Source: CAD feature listing. Evaluate the final solid. Frame: model axes, mm. A direction names the side the tool comes from. Round coordinates to 2 decimals unless told otherwise and drop trailing zeros. Order: outer loops, then holes, each group sorted by start corner. A loop starts at its lowest first (then second) coordinate and runs counter-clockwise, first axis right, second up. Notation, with made-up numbers: M 13.25,55.25 L 22.25,55.25 A8 ccw 22.25,60.25 Z; hole C 47.25,41.5 d7. An arc over 180 degrees is marked long. Answer in a Markdown table with one row per item. Add a question column.
```python
from build123d import *

# Parameters (mm, degrees)
SKETCH1_W                   = 30
SKETCH1_H                   = 30
BOSS_EXTRUDE1_DEPTH         = 5
SKETCH2_W                   = 1
SKETCH2_H                   = 30
BOSS_EXTRUDE2_DEPTH         = 4
LPATTERN1_COUNT             = 2
LPATTERN1_PITCH             = 10
CIRPATTERN1_COUNT           = 2
CIRPATTERN1_ANGLE           = 90
CIRPATTERN1_COPY_1_SKETCH_W = 1
CIRPATTERN1_COPY_1_SKETCH_H = 30
CIRPATTERN1_COPY_1_DEPTH    = 4
CUT_EXTRUDE2_DEPTH          = 22.794494718
CUT_EXTRUDE2_DEPTH_BACK     = 22.794494718
SKETCH4_R                   = 5
SKETCH8_W                   = 30
SKETCH8_H                   = 30
BOSS_EXTRUDE3_DEPTH         = 5
CUT_EXTRUDE3_DEPTH          = 5


# Read off the part's stored shape, not the designer's step: Cut-Extrude3
with BuildPart() as part:
    # Sketch1 → Boss-Extrude1 (new body)
    with BuildSketch(Plane(origin=(0, 0, 0), x_dir=(1, 0, 0), z_dir=(0, 1, 0))):
        Rectangle(SKETCH1_W, SKETCH1_H)
    extrude(amount=BOSS_EXTRUDE1_DEPTH)

    # Sketch2 → Boss-Extrude2 (add)
    with BuildSketch(Plane(origin=(0, 5, 0), x_dir=(1, 0, 0), z_dir=(0, 1, 0))):
        with Locations((-5, 0)):
            Rectangle(SKETCH2_W, SKETCH2_H)
    boss_extrude2 = extrude(amount=BOSS_EXTRUDE2_DEPTH)

    # LPattern1: Boss-Extrude2 ×2
    with Locations(*[(i * LPATTERN1_PITCH, 0, 0) for i in range(1, LPATTERN1_COUNT)]):
        add(boss_extrude2)

    # CirPattern1: Boss-Extrude2 ×2 about axis
    cirpattern1_axis = Axis((0, 5, 0), (0, 1, 0))
    for i in range(1, CIRPATTERN1_COUNT):
        add(boss_extrude2.rotate(cirpattern1_axis, i * CIRPATTERN1_ANGLE / (CIRPATTERN1_COUNT - 1)))

    # CirPattern1 copy 1 sketch → CirPattern1 copy 1 (add)
    with BuildSketch(Plane(origin=(0, 5, -10), x_dir=(0, 0, -1), z_dir=(0, 1, 0))):
        with Locations((-5, 0)):
            Rectangle(CIRPATTERN1_COPY_1_SKETCH_W, CIRPATTERN1_COPY_1_SKETCH_H)
    extrude(amount=CIRPATTERN1_COPY_1_DEPTH)

    # Sketch4 → Cut-Extrude2 (cut, two sides: drawn at the far end of the back side and taken through both)
    with BuildSketch(Plane(origin=(0, 5, 0), x_dir=(1, 0, 0), z_dir=(0, 1, 0)).offset(-CUT_EXTRUDE2_DEPTH_BACK)):
        with Locations(Location((0, 0, 0), (0, 0, 270))):
            Circle(SKETCH4_R)
    extrude(amount=CUT_EXTRUDE2_DEPTH + CUT_EXTRUDE2_DEPTH_BACK, mode=Mode.SUBTRACT)

    # Sketch8 → Boss-Extrude3 (add)
    with BuildSketch(Plane.XZ):
        Rectangle(SKETCH8_W, SKETCH8_H)
    extrude(amount=BOSS_EXTRUDE3_DEPTH)

    # Cut-Extrude3 outline → Cut-Extrude3 (cut)
    with BuildSketch(Plane.XZ):
        with BuildLine():
            ThreePointArc((7.62, 8.626), (7.173630735, 9.703630735), (6.096, 10.15))
            Line((6.096, 10.15), (-6.096, 10.15))
            ThreePointArc((-6.096, 10.15), (-7.173630735, 9.703630735), (-7.62, 8.626))
            Line((-7.62, 8.626), (-7.62, -8.626))
            ThreePointArc((-7.62, -8.626), (-7.173630735, -9.703630735), (-6.096, -10.15))
            Line((-6.096, -10.15), (6.096, -10.15))
            ThreePointArc((6.096, -10.15), (7.173630735, -9.703630735), (7.62, -8.626))
            Line((7.62, -8.626), (7.62, 8.626))
        make_face()
    extrude(amount=CUT_EXTRUDE3_DEPTH, mode=Mode.SUBTRACT)


solid = part.part
```
(1) Pin query (flat end, axial travel): pin 1 (0.7 mm diameter, centred on y = 6.5, z = -3.5, fed in from -X); pin 2 (0.7 mm diameter, centred on y = 6.5, z = -3.5, fed in from +X); pin 3 (4.5 mm diameter, centred on x = -9.5, z = -1, fed in from +Y). Return the tip coordinate at first contact, or that it passes through.
(2) Access query for faces 4 (the face through (10, 5, -10)), 5 (the face through (7.162, -2.465, -9.715)), 6 (the face through (-5.5, 7, 0)), 7 (the face through (-4.5, 7, -10)). Directions: +Z, -Z, +X, -X, +Y, -Y. A direction counts if a zero-diameter tool reaches every point of the face in a straight line with its end or side. Return the directions, or none.
(3) Line query: line 1 (X direction, y = 6.25, z = 0); line 2 (Z direction, x = -2.5, y = -0.5); line 3 (Z direction, x = 0, y = 2). Output: solid intervals per line, ascending. Write a range as from..to.
(4) Cut plane B-B (x = 0). Return loops of the section in (y, z), and give its area (4 significant figures).
(5) Cut plane D-D (x = 10). Return loops of the section in (y, z).
(6) Draft query along Z for faces 1 (the face through (4.5, 7, 10)), 2 (the face through (-3, 7, -4.5)), 3 (the face through (10, 7, -5.5)). Return one class per face: +Z half, -Z half, draft (parallel to the pull), parting line (faces both ways), or undercut.
(7) Cut plane C-C (y = -1.25). Return loops of the section in (x, z).
(8) Cut plane A-A (z = 0). Return loops of the section in (x, y).
Answer list:
| question | item | result |
|---|---|---|
| 1 | pin 1 | x = -5.5 |
| 1 | pin 2 | x = 5.5 |
| 1 | pin 3 | y = 5 |
| 2 | face 4 | -Z, +X, +Y |
| 2 | face 5 | -Y |
| 2 | face 6 | -X, +Y |
| 2 | face 7 | -Z, +Y |
| 3 | line 1 | -5.5..-5, 5..5.5 |
| 3 | line 2 | -15..-10.15, 10.15..15 |
| 3 | line 3 | -15..-5, 5..15 |
| 4 | outline | M -5,-15 L 5,-15 L 5,-5.5 L 9,-5.5 L 9,-5 L 0,-5 L 0,-10.15 L -5,-10.15 Z; M -5,10.15 L 0,10.15 L 0,5 L 9,5 L 9,5.5 L 5,5.5 L 5,15 L -5,15 Z |
| 4 | area | 152.5 mm² |
| 5 | outline | M -5,-15 L 5,-15 L 5,-5.5 L 9,-5.5 L 9,-4.5 L 5,-4.5 L 5,4.5 L 9,4.5 L 9,5.5 L 5,5.5 L 5,15 L -5,15 Z |
| 6 | face 1 | draft |
| 6 | face 2 | undercut |
| 6 | face 3 | -Z half |
| 7 | outline | M -15,-15 L 15,-15 L 15,15 L -15,15 Z; hole M -7.62,-8.63 A1.52 ccw -6.1,-10.15 L 6.1,-10.15 A1.52 ccw 7.62,-8.63 L 7.62,8.63 A1.52 ccw 6.1,10.15 L -6.1,10.15 A1.52 ccw -7.62,8.63 Z |
| 8 | outline | M -15,-5 L -7.62,-5 L -7.62,0 L -5,0 L -5,9 L -5.5,9 L -5.5,5 L -15,5 Z; M 5,0 L 7.62,0 L 7.62,-5 L 15,-5 L 15,5 L 5.5,5 L 5.5,9 L 5,9 Z |
